from build123d import *

# Parameters (mm, degrees)
F1_DEPTH = 63.5
F2_W     = 25.4
F2_H     = 50.8
F3_DEPTH = 104.14
F5_DEPTH = 19.05


with BuildPart() as f1:
    # F0 (on Front) → F1 (new body)
    with BuildSketch(Plane.XZ):
        Polygon((-51.261814, 60.08761), (-50.338179, -16.11239), (51.261821, -16.11239), (51.261821, 60.08761), align=None)
    extrude(amount=F1_DEPTH)

    # F2 (on face) → F3 (cut)
    with BuildSketch(Plane.YZ.offset(51.261821)):
        with Locations((-50.8, 34.68761)):
            Rectangle(F2_W, F2_H)
    extrude(amount=-F3_DEPTH, mode=Mode.SUBTRACT)

    # F4 (on face) → F5 (cut)
    with BuildSketch(Plane.XZ.offset(38.1)):
        Polygon((24.941918, 60.08761), (-25.861814, 60.08761), (-25.392567, 21.374697), (25.403702, 21.990409), align=None)
    extrude(amount=-F5_DEPTH, mode=Mode.SUBTRACT)


solid = f1.part
Input: part model. Units: mm. Frame: model coordinates. A direction names the side the tool comes from. Round coordinates to 2 decimals unless told otherwise and drop trailing zeros. Write each loop counter-clockwise with the first axis right and the second up, starting at its lowest first coordinate (ties: lowest second). Pieces come first, ordered by that corner, then holes.
1) Cut plane A-A (y = -32). Return the cut outline in (x, z), then the cut area to 3 significant figures.
2) Cut plane C-C (x = 32.5). Return the cut outline in (y, z).
3) Reachability of faces 1 (the flat face through (1, -51, 9.288)), 2 (the flat face through (0, -63.5, -3)), 3 (the flat face through (-1, -19.05, 41)) from +Z, -Z, +X, -X, +Y, -Y: full face, straight path, thin tool, end or side. Return the list, or none.
4) Draft query along Z for faces 4 (the flat face through (1, -38.1, 17)), 5 (the flat face through (1, -15, 60.088)), 6 (the flat face through (0, -31, -16.112)). Return one class per face: pulls with the +Z half, pulls with the -Z half, needs draft (parallel to the pull), parting line crosses it, or undercut.
5) Cut plane D-D (y = -42). Return the cut outline in (x, z).
6) Ray query, L1, parallel to Z at x = 4, y = -51; L2, parallel to Y at x = -16, z = 35; L3, parallel to Y at x = 38, z = 14. Return the intervals inside material, ascending.
7) Cut plane B-B (x = 16). Return the cut outline in (y, z), then the cut area to 3 significant figures.
8) Contact query for flat-ended pins moving along their axis: P1, Ø8, axis at x = -40, z = 39.5, coming from the -Y side; P2, Ø1.5, axis at x = 10, z = 52, coming from the +Y side; P3, Ø8, axis at y = -34.5, z = 23, coming from the -X side. Output: stop coordinate, or through.
Geometry says:
1. outline: (-51.26, 60.09) - (-50.34, -16.11) - (51.26, -16.11) - (51.26, 60.09) - (24.94, 60.09) - (25.4, 21.99) - (-25.39, 21.37) - (-25.86, 60.09) - close
1. area: 5,830 mm2
2. outline: (-63.5, -16.11) - (0, -16.11) - (0, 60.09) - (-38.1, 60.09) - (-38.1, 9.29) - (-63.5, 9.29) - close
3. face 1: +Z, +X, -X, -Y
3. face 2: +Z, -Z, +X, -X, -Y
3. face 3: +Z, -Y
4. face 4: needs draft
4. face 5: pulls with the +Z half
4. face 6: pulls with the -Z half
5. outline: (-50.65, 9.29) - (-50.34, -16.11) - (51.26, -16.11) - (51.26, 9.29) - close
6. L1: z = -16.11 to 9.29
6. L2: y = -19.05 to 0
6. L3: y = -38.1 to 0
7. outline: (-63.5, -16.11) - (0, -16.11) - (0, 60.09) - (-19.05, 60.09) - (-19.05, 21.88) - (-38.1, 21.88) - (-38.1, 9.29) - (-63.5, 9.29) - close
7. area: 2,820 mm2
8. P1: stops at y = -38.1
8. P2: stops at y = 0
8. P3: stops at x = -50.86
